```python
from build123d import *

# Parameters (mm, degrees)
F0_W     = 180
F0_H     = 224
F0_R     = 1.5
F0_R_2   = 32.5
F1_DEPTH = 10
F3_DEPTH = 5


with BuildPart() as f1:
    # F0 (on Top) → F1 (new body)
    with BuildSketch(Plane.XY):
        Rectangle(F0_W, F0_H)
        with Locations((-50, -100)):
            Circle(F0_R, mode=Mode.SUBTRACT)
        with Locations((-82.5, -20)):
            Circle(F0_R, mode=Mode.SUBTRACT)
        with Locations((50, -100)):
            Circle(F0_R, mode=Mode.SUBTRACT)
        with Locations((82.5, -20)):
            Circle(F0_R, mode=Mode.SUBTRACT)
        with Locations((-82.5, 20)):
            Circle(F0_R, mode=Mode.SUBTRACT)
        with Locations((-50, 100)):
            Circle(F0_R, mode=Mode.SUBTRACT)
        Polygon((75, -53.7867965644), (75, -75), (75, -88), (66.7867965644, -88), (-66.7867965644, -88), (-75, -88), (-75, -75), (-75, -53.7867965644), (-75, 53.7867965644), (-75, 75), (-75, 88), (-66.7867965644, 88), (66.7867965644, 88), (75, 88), (75, 75), (75, 53.7867965644), align=None, mode=Mode.SUBTRACT)
        with Locations((82.5, 20)):
            Circle(F0_R, mode=Mode.SUBTRACT)
        with Locations((50, 100)):
            Circle(F0_R, mode=Mode.SUBTRACT)
        with BuildLine():
            Line((-53.7867965644, 75), (-66.7867965644, 88))
            Line((-66.7867965644, 88), (-75, 88))
            Line((-75, 88), (-75, 75))
            Line((-75, 75), (-75, 53.7867965644))
            Line((-75, 53.7867965644), (-44.3334456259, 23.1202421903))
            ThreePointArc((-44.3334456259, 23.1202421903), (-35.3553390593, 35.3553390593), (-23.1202421903, 44.3334456259))
            Line((-23.1202421903, 44.3334456259), (-53.7867965644, 75))
        make_face()
        with Locations((-67.1751442127, 53.033008589)):
            Circle(F0_R, mode=Mode.SUBTRACT)
        with Locations((-53.033008589, 67.1751442127)):
            Circle(F0_R, mode=Mode.SUBTRACT)
        with BuildLine():
            ThreePointArc((23.1202421903, -44.3334456259), (35.3553390593, -35.3553390593), (44.3334456259, -23.1202421903))
            ThreePointArc((44.3334456259, -23.1202421903), (48.5627031851, -11.9022627829), (50, 0))
            ThreePointArc((50, 0), (48.5627031851, 11.9022627829), (44.3334456259, 23.1202421903))
            ThreePointArc((44.3334456259, 23.1202421903), (40.3112887415, 29.5803989155), (35.3553390593, 35.3553390593))
            ThreePointArc((35.3553390593, 35.3553390593), (29.5803989155, 40.3112887415), (23.1202421903, 44.3334456259))
            ThreePointArc((23.1202421903, 44.3334456259), (11.9022627829, 48.5627031851), (0, 50))
            ThreePointArc((0, 50), (-11.9022627829, 48.5627031851), (-23.1202421903, 44.3334456259))
            ThreePointArc((-23.1202421903, 44.3334456259), (-35.3553390593, 35.3553390593), (-44.3334456259, 23.1202421903))
            ThreePointArc((-44.3334456259, 23.1202421903), (-48.5627031851, 11.9022627829), (-50, 0))
            ThreePointArc((-50, 0), (-48.5627031851, -11.9022627829), (-44.3334456259, -23.1202421903))
            ThreePointArc((-44.3334456259, -23.1202421903), (-35.3553390593, -35.3553390593), (-23.1202421903, -44.3334456259))
            ThreePointArc((-23.1202421903, -44.3334456259), (-11.9022627829, -48.5627031851), (0, -50))
            ThreePointArc((0, -50), (11.9022627829, -48.5627031851), (23.1202421903, -44.3334456259))
        make_face()
        with Locations((-24.7487373415, -38.8908729653)):
            Circle(F0_R, mode=Mode.SUBTRACT)
        with Locations((-38.8908729653, -24.7487373415)):
            Circle(F0_R, mode=Mode.SUBTRACT)
        with Locations((24.7487373415, -38.8908729653)):
            Circle(F0_R, mode=Mode.SUBTRACT)
        with Locations((38.8908729653, -24.7487373415)):
            Circle(F0_R, mode=Mode.SUBTRACT)
        with Locations((-38.8908729653, 24.7487373415)):
            Circle(F0_R, mode=Mode.SUBTRACT)
        with Locations((-24.7487373415, 38.8908729653)):
            Circle(F0_R, mode=Mode.SUBTRACT)
        Circle(F0_R_2, mode=Mode.SUBTRACT)
        with Locations((38.8908729653, 24.7487373415)):
            Circle(F0_R, mode=Mode.SUBTRACT)
        with Locations((24.7487373415, 38.8908729653)):
            Circle(F0_R, mode=Mode.SUBTRACT)
        with BuildLine():
            Line((44.3334456259, 23.1202421903), (75, 53.7867965644))
            Line((75, 53.7867965644), (75, 75))
            Line((75, 75), (75, 88))
            Line((75, 88), (66.7867965644, 88))
            Line((66.7867965644, 88), (53.7867965644, 75))
            Line((53.7867965644, 75), (23.1202421903, 44.3334456259))
            ThreePointArc((23.1202421903, 44.3334456259), (29.5803989155, 40.3112887415), (35.3553390593, 35.3553390593))
            ThreePointArc((35.3553390593, 35.3553390593), (40.3112887415, 29.5803989155), (44.3334456259, 23.1202421903))
        make_face()
        with Locations((67.1751442127, 53.033008589)):
            Circle(F0_R, mode=Mode.SUBTRACT)
        with Locations((53.033008589, 67.1751442127)):
            Circle(F0_R, mode=Mode.SUBTRACT)
        with BuildLine():
            Line((75, -88), (75, -75))
            Line((75, -75), (75, -53.7867965644))
            Line((75, -53.7867965644), (44.3334456259, -23.1202421903))
            ThreePointArc((44.3334456259, -23.1202421903), (35.3553390593, -35.3553390593), (23.1202421903, -44.3334456259))
            Line((23.1202421903, -44.3334456259), (53.7867965644, -75))
            Line((53.7867965644, -75), (66.7867965644, -88))
            Line((66.7867965644, -88), (75, -88))
        make_face()
        with Locations((53.033008589, -67.1751442127)):
            Circle(F0_R, mode=Mode.SUBTRACT)
        with Locations((67.1751442127, -53.033008589)):
            Circle(F0_R, mode=Mode.SUBTRACT)
        with BuildLine():
            Line((-75, -88), (-66.7867965644, -88))
            Line((-66.7867965644, -88), (-23.1202421903, -44.3334456259))
            ThreePointArc((-23.1202421903, -44.3334456259), (-35.3553390593, -35.3553390593), (-44.3334456259, -23.1202421903))
            Line((-44.3334456259, -23.1202421903), (-75, -53.7867965644))
            Line((-75, -53.7867965644), (-75, -75))
            Line((-75, -75), (-75, -88))
        make_face()
        with Locations((-53.033008589, -67.1751442127)):
            Circle(F0_R, mode=Mode.SUBTRACT)
        with Locations((-67.1751442127, -53.033008589)):
            Circle(F0_R, mode=Mode.SUBTRACT)
    extrude(amount=F1_DEPTH)

    # F2 (on face) → F3 (cut)
    with BuildSketch(Plane.XY.offset(10)):
        with BuildLine():
            Line((-90, 97.0710678119), (-90, 82.9289321881))
            Line((-90, 82.9289321881), (-26.2429115617, 19.1718437498))
            ThreePointArc((-26.2429115617, 19.1718437498), (-22.9809703886, 22.9809703886), (-19.1718437498, 26.2429115617))
            Line((-19.1718437498, 26.2429115617), (-90, 97.0710678119))
        make_face()
        with BuildLine():
            Line((90, 97.0710678119), (19.1718437498, 26.2429115617))
            ThreePointArc((19.1718437498, 26.2429115617), (22.9809703886, 22.9809703886), (26.2429115617, 19.1718437498))
            Line((26.2429115617, 19.1718437498), (90, 82.9289321881))
            Line((90, 82.9289321881), (90, 97.0710678119))
        make_face()
        with BuildLine():
            ThreePointArc((26.2429115617, -19.1718437498), (22.9809703886, -22.9809703886), (19.1718437498, -26.2429115617))
            Line((19.1718437498, -26.2429115617), (90, -97.0710678119))
            Line((90, -97.0710678119), (90, -82.9289321881))
            Line((90, -82.9289321881), (26.2429115617, -19.1718437498))
        make_face()
        with BuildLine():
            Line((-26.2429115617, -19.1718437498), (-90, -82.9289321881))
            Line((-90, -82.9289321881), (-90, -97.0710678119))
            Line((-90, -97.0710678119), (-19.1718437498, -26.2429115617))
            ThreePointArc((-19.1718437498, -26.2429115617), (-22.9809703886, -22.9809703886), (-26.2429115617, -19.1718437498))
        make_face()
    extrude(amount=-F3_DEPTH, mode=Mode.SUBTRACT)


solid = f1.part
```
Build history of the part. All positions in model axes, mm. A direction names the side the tool comes from. Coordinates: 2 decimals unless noted, no trailing zeros. Order: outer loops, then holes, each group sorted by start corner. A loop starts at its lowest first (then second) coordinate and runs counter-clockwise, first axis right, second up. Notation, with made-up numbers: M -1.5,65.5 L 11.5,65.5 A19 cw 11.5,87.5 Z; hole C 56.25,3.5 d1. An arc over 180 degrees is marked long. One line per question, with ' | ' between items. Start each with the question number.
1. Cut at D-D (z = 2.25). Count the separate pieces of the cut face and the enclosed holes in it, plus the area to 3 significant figures.
2. Cut at C-C (y = -76.5). Write the cut outline in (x, z).
3. Cut at B-B (x = 71.5). Write the cut outline in (y, z).
4. Cut at A-A (y = -3.5). Write the cut outline in (x, z).
5. Mould opens along Y. For faces 4 (the face through (-58.57, 51.5, 7.54)), 5 (the face through (-1, -97, 10)), 6 (the face through (59.452, 38.239, 4.93)), 7 (the face through (-1, 112, 5)) say: +Y half, -Y half, draft (parallel to the pull), parting line (faces both ways), or undercut.
6. Wall check: line 1 along Y through (x, z) = (-82.5, 3.5); line 2 along Y through (x, z) = (1.5, 9.25); line 3 along X through (y, z) = (-100, 5.25). Give the ranges that are in metal, low to high. Write a range as [from, to].
7. Tool access for faces 1 (the face through (90, -2, 5)), 2 (the face through (1, -88, 5)), 3 (the face through (58.57, -51.5, 7.54)): list every direction of +Z, -Z, +X, -X, +Y, -Y with a clear straight run to the whole face (end or side of a thin tool).
The answers:
1) separate pieces: 1 | enclosed holes: 29 | area: 25,000 mm2
2) outline: M -90,0 L -55.29,0 L -55.29,10 L -69.43,10 L -69.43,5 L -83.57,5 L -83.57,10 L -90,10 Z; M 55.29,0 L 90,0 L 90,10 L 83.57,10 L 83.57,5 L 69.43,5 L 69.43,10 L 55.29,10 Z
3) outline: M -112,0 L -50.29,0 L -50.29,10 L -64.43,10 L -64.43,5 L -78.57,5 L -78.57,10 L -112,10 Z; M 50.29,0 L 112,0 L 112,10 L 78.57,10 L 78.57,5 L 64.43,5 L 64.43,10 L 50.29,10 Z
4) outline: M -90,0 L -75,0 L -75,10 L -90,10 Z; M -49.88,0 L -32.31,0 L -32.31,10 L -49.88,10 Z; M 32.31,0 L 49.88,0 L 49.88,10 L 32.31,10 Z; M 75,0 L 90,0 L 90,10 L 75,10 Z
5) face 4: undercut | face 5: draft | face 6: undercut | face 7: +Y half
6) line 1: y = [-112, -21.5], [-18.5, 18.5], [21.5, 112] | line 2: y = [-112, -88], [-49.98, -32.47], [32.47, 49.98], [88, 112] | line 3: x = [-90, -51.5], [-48.5, 48.5], [51.5, 90]
7) face 1: +Z, -Z, +X, +Y, -Y | face 2: +Z, -Z | face 3: +Z
